Input: part model. Units: mm. Frame: model coordinates. A direction names the side the tool comes from. Give positions to 0.01 mm unless a question says otherwise; leave off trailing zeros. Loops run counter-clockwise (first coordinate to the right, second up) from the corner with the lowest first, then second, coordinate; pieces in that order, holes last. Notation, with made-up numbers: (-34.5, -21) - (20.5, -21) arc R13 cw to (20.5, -6) - close; hole circle Ø2 at (51.25, 75.25). An arc over 180 degrees is marked (long way). One line per item, written item: value.
from build123d import *

# Parameters (mm, degrees)
F0_W     = 12.7
F0_H     = 12.7
F1_DEPTH = 12.7
F2_DEPTH = 12.7


with BuildPart() as f1:
    # F0 (on Front) → F1 (new body)
    with BuildSketch(Plane.XZ):
        with Locations((18.5406431556, 58.970926)):
            Rectangle(F0_W, F0_H)
        with BuildLine():
            Line((12.1906431556, 52.620926), (12.1906431556, 65.320926))
            add(Edge.make_bspline(
                [(12.1906431556, 65.320926), (1.6408012652, 47.6242484273), (-15.7682649232, 18.4216656416), (-32.2303568983, 10.6729982106), (-38.7164705157, 7.62)],
                knots=[0, 0, 0, 0, 0.6059970004, 1, 1, 1, 1], degree=3))
            Line((-38.7164705157, 7.62), (-63.4810701013, 7.62))
            ThreePointArc((-63.4810701013, 7.62), (-67.2910701013, 3.81), (-63.4810701013, 0))
            Line((-63.4810701013, 0), (-38.7164705157, 0))
            add(Edge.make_bspline(
                [(12.1906431556, 52.620926), (3.8448232521, 37.5782991027), (-10.2312518477, 10.0416995234), (-31.0323794757, 3.2870267288), (-38.7164705157, 0)],
                knots=[0, 0, 0, 0, 0.5675080648, 1, 1, 1, 1], degree=3))
        make_face()
    extrude(amount=F1_DEPTH)

    # F0 (on Front) → F2 (join)
    with BuildSketch(Plane.XZ):
        with Locations((18.5406431556, 58.970926)):
            Rectangle(F0_W, F0_H)
        with BuildLine():
            Line((12.1906431556, 52.620926), (12.1906431556, 65.320926))
            add(Edge.make_bspline(
                [(12.1906431556, 65.320926), (1.6408012652, 47.6242484273), (-15.7682649232, 18.4216656416), (-32.2303568983, 10.6729982106), (-38.7164705157, 7.62)],
                knots=[0, 0, 0, 0, 0.6059970004, 1, 1, 1, 1], degree=3))
            Line((-38.7164705157, 7.62), (-63.4810701013, 7.62))
            ThreePointArc((-63.4810701013, 7.62), (-67.2910701013, 3.81), (-63.4810701013, 0))
            Line((-63.4810701013, 0), (-38.7164705157, 0))
            add(Edge.make_bspline(
                [(12.1906431556, 52.620926), (3.8448232521, 37.5782991027), (-10.2312518477, 10.0416995234), (-31.0323794757, 3.2870267288), (-38.7164705157, 0)],
                knots=[0, 0, 0, 0, 0.5675080648, 1, 1, 1, 1], degree=3))
        make_face()
    extrude(amount=F2_DEPTH)


solid = f1.part
Item 1: Material intervals for L1, parallel to Z at x = 14, y = -2; L2, parallel to Z at x = -43.5, y = -1.5; L3, parallel to X at y = -6, z = 46.5, sorted ascending.
Verdict:
L1: z = 52.62 to 65.32
L2: z = 0 to 7.62
L3: x = 0.77 to 8.82
Item 2: Access query for faces 1 (the face through (-51, -6, 7.62)), 2 (the face through (18, -6, 52.621)), 3 (the face through (-67.29, -6.26, 3.89)). Directions: +Z, -Z, +X, -X, +Y, -Y. A direction counts if a zero-diameter tool reaches every point of the face in a straight line with its end or side. Return the directions, or none.
Verdict:
face 1: +Z, -X, +Y, -Y
face 2: -Z, +X, +Y, -Y
face 3: -X, +Y, -Y
Item 3: Pin query (flat end, axial travel): P1, Ø4, axis at y = -8, z = 17, coming from the +X side; P2, Ø1.5, axis at x = -25, y = -3, coming from the +Z side; P3, Ø5, axis at x = -1.5, y = -5.5, coming from the -Z side. Return the tip coordinate at first contact, or that it passes through.
Verdict:
P1: stops at x = -8.55
P2: stops at z = 15.75
P3: stops at z = 25.01
Item 4: Section B-B, the plane x = -62. Output: boundary loops of the cut face in (y, z).
Verdict:
outline: (-12.7, 0) - (0, 0) - (0, 7.62) - (-12.7, 7.62) - close
Item 5: Section A-A, the plane x = 14. Output: boundary loops of the cut face in (y, z), and give its area (3 significant figures).
Verdict:
outline: (-12.7, 52.62) - (0, 52.62) - (0, 65.32) - (-12.7, 65.32) - close
area: 161 mm^2
